from build123d import *

# Parameters (mm, degrees)
SKETCH1_R           = 0.875
BOSS_EXTRUDE1_DEPTH = 3
CHAMFER1_SIZE       = 5
BOSS_EXTRUDE2_DEPTH = 5
SKETCH2_R           = 1.5
CUT_EXTRUDE1_DEPTH  = 4
CHAMFER2_SIZE       = 1


with BuildPart() as part:
    # Sketch1 → Boss-Extrude1 (new body)
    with BuildSketch(Plane.XY):
        Polygon((4.9, 3), (4.9, 1.5), (7.5, 1.5), (7.5, 0), (-7.5, 0), (-7.5, 1.5), (-4.9, 1.5), (-4.9, 3), align=None)
        Polygon((4.9, 3), (-4.9, 3), (-11, 3), (-11, 27), (-7, 27), (-7, 7), (7, 7), (7, 27), (11, 27), (11, 3), align=None)
        with Locations((-9, 14)):
            Circle(SKETCH1_R, mode=Mode.SUBTRACT)
        with Locations((9, 14)):
            Circle(SKETCH1_R, mode=Mode.SUBTRACT)
        with Locations((9, 25)):
            Circle(SKETCH1_R, mode=Mode.SUBTRACT)
        with Locations((-9, 25)):
            Circle(SKETCH1_R, mode=Mode.SUBTRACT)
    extrude(amount=BOSS_EXTRUDE1_DEPTH)

    # Chamfer1
    chamfer1_edges = [part.edges().sort_by_distance(p)[0] for p in [
        (-11, 3, 1.5),
        (-7, 7, 1.5),
        (7, 7, 1.5),
        (11, 3, 1.5),
    ]]
    chamfer(chamfer1_edges, length=CHAMFER1_SIZE)

    # Sketch1_4 → Boss-Extrude2 (add)
    with BuildSketch(Plane.XY):
        Polygon((4.9, 3), (4.9, 1.5), (7.5, 1.5), (7.5, 0), (-7.5, 0), (-7.5, 1.5), (-4.9, 1.5), (-4.9, 3), align=None)
    extrude(amount=-BOSS_EXTRUDE2_DEPTH)

    # Sketch2 → Cut-Extrude1 (cut, through all)
    with BuildSketch(Plane(origin=(0, 3, 0), x_dir=(1, 0, 0), z_dir=(0, 1, 0))):
        with Locations((0, 3)):
            Circle(SKETCH2_R)
    extrude(amount=-CUT_EXTRUDE1_DEPTH, mode=Mode.SUBTRACT)

    # Chamfer2
    chamfer2_edges = [part.edges().sort_by_distance(p)[0] for p in [
        (0, 3, 0),
    ]]
    chamfer(chamfer2_edges, length=CHAMFER2_SIZE)


solid = part.part
Read the model definition and answer for the solid it produces. Units are mm, in the model's axes. A direction names the side the tool comes from. Round coordinates to 2 decimals unless told otherwise and drop trailing zeros. Loops run counter-clockwise (first coordinate to the right, second up) from the corner with the lowest first, then second, coordinate; pieces in that order, holes last. Notation, with made-up numbers: (-29.75, 53) - (-25.75, 53) arc R9 ccw to (-25.75, 69) - close; hole circle Ø4 at (54.25, 68). An arc over 180 degrees is marked (long way). One line per question, with ' | ' between items. Start each with the question number.
Q1. Section A-A on y = 12.5 is taken. Give the vertices of the cut face in (x, z), plus the area to 3 significant figures.
Q2. Find the intervals of material crossed by L1, parallel to Y at x = -9, z = 1.25 (3 decimals); L2, parallel to Z at x = 0, y = 2.2; L3, parallel to Y at x = 1.5, z = -2.5, in increasing order.
Q3. Section B-B on x = -9 is taken. Give the vertices of the cut face in (y, z) (3 decimals), plus the area to 3 significant figures.
Q4. Section C-C on y = 25 is taken. Give the vertices of the cut face in (x, z) (3 decimals).
Q5. For faces 4 (the flat face through (-7.5, 1, -1)), 5 (the flat face through (-6, 1.5, -1)), 6 (the flat face through (7.5, 1, -1)), determine the directions among +Z, -Z, +X, -X, +Y, -Y from which every point of the face is accessible in a straight line to the end or side of a thin tool.
Q6. For a pull along Z with two mould halves and no side action, classify faces 1 (the flat face through (9, 6, 1)), 2 (the cylindrical face through (-0.325, 1.521, -1.536)), 3 (the flat face through (3, 7, 0)) as +Z half, -Z half, draft (parallel to the pull), parting line (faces both ways), or undercut.
Q7. Flat-ended cylindrical pins translate along their axes: pin 1 (1.4 mm diameter, centred on x = 9, y = 25, fed in from +Z); pin 2 (0.8 mm diameter, centred on y = 2.5, z = -2, fed in from +X); pin 3 (0.9 mm diameter, centred on x = 0, z = 1, fed in from +Y); pin 4 (1.5 mm diameter, centred on x = 7.5, y = 9, fed in from -Z). Find the tip coordinate at first contact, or state that the pin passes through.
Q8. Section D-D on z = -3 is taken. Give the vertices of the cut face in (x, y).
Established:
1) outline: (-11, 0) - (-7, 0) - (-7, 3) - (-11, 3) - close; (7, 0) - (11, 0) - (11, 3) - (7, 3) - close | area: 24.0 mm²
2) L1: 6 to 13.125, 14.875 to 24.125, 25.875 to 27 | L2: -5 to -4.5, -1.5 to 3 | L3: 0 to 3
3) outline: (6, 0) - (13.125, 0) - (13.125, 3) - (6, 3) - close; (14.875, 0) - (24.125, 0) - (24.125, 3) - (14.875, 3) - close; (25.875, 0) - (27, 0) - (27, 3) - (25.875, 3) - close | area: 52.5 mm²
4) outline: (-11, 0) - (-9.875, 0) - (-9.875, 3) - (-11, 3) - close; (-8.125, 0) - (-7, 0) - (-7, 3) - (-8.125, 3) - close; (7, 0) - (8.125, 0) - (8.125, 3) - (7, 3) - close; (9.875, 0) - (11, 0) - (11, 3) - (9.875, 3) - close
5) face 4: +Z, -Z, -X, -Y | face 5: +Z, -Z, -X | face 6: +Z, -Z, +X, -Y
6) face 1: draft | face 2: undercut | face 3: -Z half
7) pin 1: through | pin 2: x = 4.9 | pin 3: y = 7 | pin 4: z = 0
8) outline: (-7.5, 0) - (-1.5, 0) - (-1.5, 3) - (-4.9, 3) - (-4.9, 1.5) - (-7.5, 1.5) - close; (1.5, 0) - (7.5, 0) - (7.5, 1.5) - (4.9, 1.5) - (4.9, 3) - (1.5, 3) - close
